Part print with two shaded views. Sizes in mm from the minimum x, y, z corner. Coordinates: 2 decimals unless noted, no trailing zeros. Write each loop counter-clockwise with the first axis right and the second up, starting at its lowest first coordinate (ties: lowest second). Pieces come first, ordered by that corner, then holes.
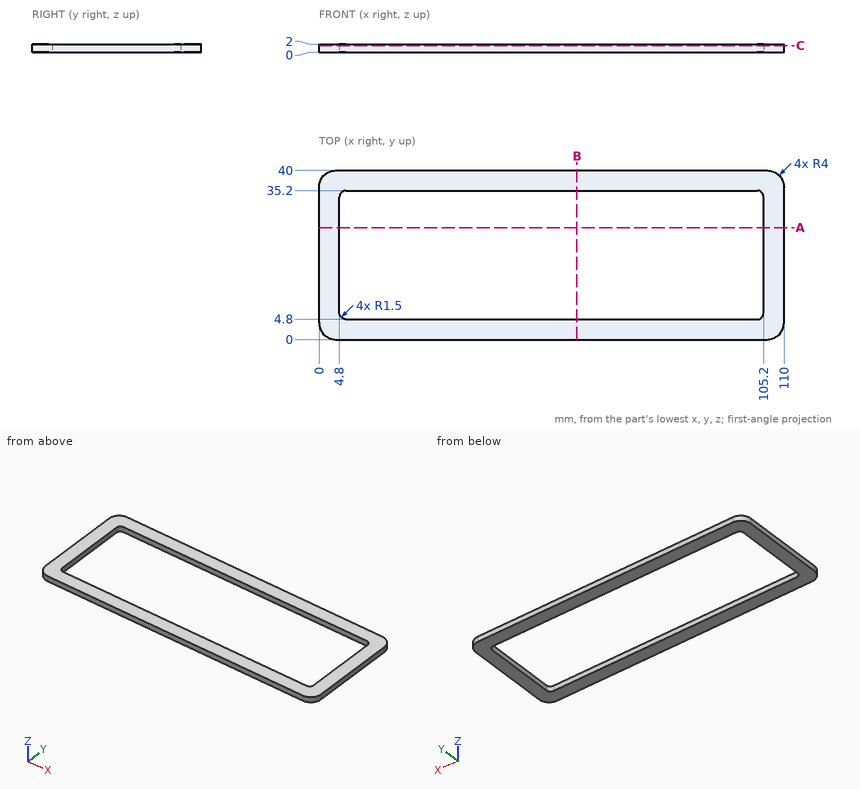
(1) Slice it at C-C, the plane z = 1.6. List the corners of the cut face in (x, y).
(2) Probe L1, parallel to Y at x = 102.5, z = 0.75; L2, parallel to X at y = 29, z = 0.4. List the from-to ranges inside material, lowest first.
(3) Slice it at B-B, the plane x = 61. List the corners of the cut face in (y, z), and give its area (3 significant figures).
(4) Slice it at A-A, the plane y = 26.5. List the corners of the cut face in (x, z), and give its area (3 significant figures).
Results:
1. outline: (0, 4) arc R4 ccw to (4, 0) - (106, 0) arc R4 ccw to (110, 4) - (110, 36) arc R4 ccw to (106, 40) - (4, 40) arc R4 ccw to (0, 36) - close; hole (4.8, 6.3) arc R1.5 ccw to (6.3, 4.8) - (103.7, 4.8) arc R1.5 ccw to (105.2, 6.3) - (105.2, 33.7) arc R1.5 ccw to (103.7, 35.2) - (6.3, 35.2) arc R1.5 ccw to (4.8, 33.7) - close
2. L1: y = 0 to 4.8, 35.2 to 40
2. L2: x = 0 to 4.8, 105.2 to 110
3. outline: (0, 0) - (4.8, 0) - (4.8, 2) - (0, 2) - close; (35.2, 0) - (40, 0) - (40, 2) - (35.2, 2) - close
3. area: 19.2 mm2
4. outline: (0, 0) - (4.8, 0) - (4.8, 2) - (0, 2) - close; (105.2, 0) - (110, 0) - (110, 2) - (105.2, 2) - close
4. area: 19.2 mm2
